Autodesk Inventor part; units mm, degrees
ref_plane "YZ Plane" through (0, 0, 0) normal (1, 0, 0) x (0, 1, 0)
ref_plane "XZ Plane" through (0, 0, 0) normal (0, 1, 0) x (-1, 0, 0)
ref_plane "XY Plane" through (0, 0, 0) normal (0, 0, 1) x (1, 0, 0)
sketch "Sketch1" plane through (0, 0, 0) normal (0, 0, 1) x (1, 0, 0)
  line L0 (-5, -2.5) -> (5, -2.5) construction
  line L1 (5, -2.5) -> (12.675, 0) construction
  line L2 (-5, -2.5) -> (-12.675, 0)
  line L3 (12.675, 0) -> (-12.675, 0) construction
  line L4 (12.675, 0) -> (12.675, 8.7) construction
  line L5 (-12.675, 0) -> (-12.675, 8.7)
  line L6 (-12.675, 8.7) -> (-4.75, 23.1)
  line L7 (-4.75, 23.1) -> (-4.75, 25.1)
  line L8 (-4.75, 25.1) -> (4.75, 25.1) construction
  line L9 (4.75, 25.1) -> (4.75, 23.1) construction
  line L10 (4.75, 23.1) -> (12.675, 8.7) construction
  line L11 (0, -9.3621) -> (0, 31.9621)
  line L12 (0, 25.1) -> (0, -2.5)
  circle A0 centre (-10.8, 4.25) radius 1.25
  line L13 (-10.8, 4.25) -> (0, 4.25) construction
  line L14 (-4.75, 25.1) -> (0, 25.1)
  line L15 (-5, -2.5) -> (0, -2.5)
  line L16 (-5.7087, 23.3464) -> (-13.6337, 8.9464)
  line L17 (-13.6337, 8.9464) -> (-13.6337, -0.696)
  line L18 (-13.6337, -0.696) -> (-5.1522, -3.4587)
  line L19 (-5.1522, -3.4587) -> (0.9587, -3.4587) construction
  line L20 (0.9587, -3.4587) -> (0.9587, 26.0587) construction
  line L21 (0.9587, 26.0587) -> (-5.7087, 26.0587) construction
  line L22 (-5.7087, 26.0587) -> (-5.7087, 23.3464)
  line L23 (0, -2.5) -> (0, -3.4587)
  line L24 (0, 25.1) -> (0, 26.0587)
  line L25 (0, -3.4587) -> (-5.1522, -3.4587)
  line L26 (0, 26.0587) -> (-5.7087, 26.0587)
  point P0 (0, 0)
  point P1 (0, 0)
  dimension "d0" = 10
  dimension "d1" = 25.35
  dimension "d2" = 2.5
  dimension "d3" = 8.7
  dimension "d4" = 27.6
  dimension "d6" = 2
  dimension "d7" = 9.5
  dimension "d42" = 2.5
  dimension "d43" = 10.8
  dimension "d44" = 6.75
  dimension "d53" = 0.9587
sketch "Sketch8" plane through (0, 0, 0) normal (0, 0, 1) x (1, 0, 0)
  line L0 (-20, 30) -> (20, 30)
  line L1 (20, 30) -> (20, -10)
  line L2 (20, -10) -> (-20, -10)
  line L3 (-20, -10) -> (-20, 30)
  point P0 (0, 0)
  point P1 (0, -10)
  dimension "d45" = 40
  dimension "d46" = 10
extrude "MainBlock" add sketch "Sketch8" against normal blind 6
extrude "CartridgeCutout" cut sketch "Sketch1" against normal blind 3
sketch "Sketch10" plane through (-10.8, 4.25, 0) normal (0, 0, 1) x (1, 0, 0)
  circle A0 centre (0, 0) radius 1.25
  circle A1 centre (0, 0) radius 1.75
  point P0 (10.8, -4.25)
  dimension "d56" = 0.5
extrude "PinHole" cut sketch "Sketch10" against normal through all contours A0 | A1
mirror "Mirror3" about plane through (0, 26.0587, 0) normal (-1, 0, 0) of "CartridgeCutout", "PinHole"
sketch "Sketch12" plane through (0, 0, -3) normal (0, 0, 1) x (1, 0, 0)
  circle A0 centre (10.8, 4.25) radius 1.75
  circle A1 centre (-10.8, 4.25) radius 1.75
  line L0 (5.7087, 26.0587) -> (-5.7087, 26.0587)
  line L1 (-5.7087, 23.3464) -> (-5.7087, 26.0587)
  line L2 (-13.6337, 8.9464) -> (-5.7087, 23.3464)
  line L3 (-13.6337, -0.696) -> (-13.6337, 8.9464)
  line L4 (-5.1522, -3.4587) -> (-13.6337, -0.696)
  line L5 (5.1522, -3.4587) -> (-5.1522, -3.4587)
  line L6 (5.1522, -3.4587) -> (13.6337, -0.696)
  line L7 (13.6337, -0.696) -> (13.6337, 8.9464)
  line L8 (13.6337, 8.9464) -> (5.7087, 23.3464)
  line L9 (5.7087, 23.3464) -> (5.7087, 26.0587)
  line L10 (-4.15, 23.6) -> (4.15, 23.6)
  line L11 (4.15, 23.6) -> (4.15, -1.4)
  line L12 (4.15, -1.4) -> (-4.15, -1.4)
  line L13 (-4.15, -1.4) -> (-4.15, 23.6)
  point P0 (0, 0)
  point P1 (0, -1.4)
  dimension "d59" = 8.3
  dimension "d60" = 25
  dimension "d61" = 1.4
extrude "Extrusion12" cut sketch "Sketch12" against normal through all contours L10 L11 L12 L13
fillet "Fillet1" radius 2 4 edges at (-20, 30, -3) (-20, -10, -3) (20, -10, -3) (20, 30, -3)
properties part number "InkjetHolder"
Here's how the part is built. I have some questions about the finished solid (model axes, mm). A direction names the side the tool comes from. Coordinates: 2 decimals unless noted, no trailing zeros. Order: outer loops, then holes, each group sorted by start corner. A loop starts at its lowest first (then second) coordinate and runs counter-clockwise, first axis right, second up. Notation, with made-up numbers: (29, 16.5) -> (86, 16.5) arc R27 cw to (86, 49.5) -> close; hole circle Ø8 at (39.5, 76.5). An arc over 180 degrees is marked (long way). Return JSON: item names as keys, results as strings.
1) If I drill on probe 1 along Y at (x, z) = (-10.8, -4.15); probe 2 along Y at (x, z) = (3.5, -0.75); probe 3 along X at (y, z) = (25, -0.25), over which ranges is the centre line in solid material (lowest first)?
Conclusion:
{"probe 1": "y = -10 to 2.5, 6 to 30", "probe 2": "y = -10 to -3.46, 26.06 to 30", "probe 3": "x = -20 to -5.71, 5.71 to 20"}
2) If we section it at C-C on z = -4.05: List the corners of the cut face in (x, y) for me.
Conclusion:
{"outline": "(-20, -8) arc R2 ccw to (-18, -10) -> (18, -10) arc R2 ccw to (20, -8) -> (20, 28) arc R2 ccw to (18, 30) -> (-18, 30) arc R2 ccw to (-20, 28) -> close; hole circle Ø3.5 at (-10.8, 4.25); hole (-4.15, -1.4) -> (4.15, -1.4) -> (4.15, 23.6) -> (-4.15, 23.6) -> close; hole circle Ø3.5 at (10.8, 4.25)"}
3) If we section it at B-B on y = 4.25: List the corners of the cut face in (x, z) for me.
Conclusion:
{"outline": "(-20, -6) -> (-12.55, -6) -> (-12.55, -3) -> (-13.63, -3) -> (-13.63, 0) -> (-20, 0) -> close; (-9.05, -6) -> (-4.15, -6) -> (-4.15, -3) -> (-9.05, -3) -> close; (4.15, -6) -> (9.05, -6) -> (9.05, -3) -> (4.15, -3) -> close; (12.55, -6) -> (20, -6) -> (20, 0) -> (13.63, 0) -> (13.63, -3) -> (12.55, -3) -> close"}
4) If we section it at D-D on z = -1.25: List the corners of the cut face in (x, y) for me.
Conclusion:
{"outline": "(-20, -8) arc R2 ccw to (-18, -10) -> (18, -10) arc R2 ccw to (20, -8) -> (20, 28) arc R2 ccw to (18, 30) -> (-18, 30) arc R2 ccw to (-20, 28) -> close; hole (-13.63, -0.7) -> (-5.15, -3.46) -> (5.15, -3.46) -> (13.63, -0.7) -> (13.63, 8.95) -> (5.71, 23.35) -> (5.71, 26.06) -> (-5.71, 26.06) -> (-5.71, 23.35) -> (-13.63, 8.95) -> close"}
5) On a 3-axis mill with a long thin cutter (end or side, diameter ignored), from which of +Z, -Z, +X, -X, +Y, -Y can I reach the whole of each face in a straight line? I mean faces 1 (the flat face through (0, 23.6, -4)), 2 (the flat face through (20, 10, -3)), 3 (the flat face through (-9.616, 16.247, -1.479)). Say none if no direction works.
Conclusion:
{"face 1": "+Z, -Z", "face 2": "+Z, -Z, +X, +Y, -Y", "face 3": "+Z"}
6) I'm going to push a flat-ended pin straight in: P1, Ø6, axis at x = 6.5, y = 14, coming from the +Z side. Where does the tip first touch, or does it pass through?
Conclusion:
{"P1": "stops at z = -3"}
7) Thinking about a two-plate mould opening in Y: for faces 4 (the cylindrical face through (-12.55, 4.33, -4.48)), 5 (the flat face through (0, 30, -3)), 6 (the cylindrical face through (19.43, -9.4, -3.04)), which applies, +Y half, -Y half, draft (parallel to the pull), parting line (faces both ways), or undercut?
Conclusion:
{"face 4": "undercut", "face 5": "+Y half", "face 6": "-Y half"}
8) If we section it at A-A on x = -0.5: List the corners of the cut face in (y, z) for me.
Conclusion:
{"outline": "(-10, -6) -> (-1.4, -6) -> (-1.4, -3) -> (-3.46, -3) -> (-3.46, 0) -> (-10, 0) -> close; (23.6, -6) -> (30, -6) -> (30, 0) -> (26.06, 0) -> (26.06, -3) -> (23.6, -3) -> close"}
